```python
from build123d import *

# Parameters (mm, degrees)
F0_W     = 101.6
F0_H     = 101.6
F1_DEPTH = 914.4
F3_DEPTH = 101.6
F4_W     = 101.6
F4_H     = 101.6
F5_DEPTH = 50.8
F6_W     = 50.8
F6_H     = 101.6
F7_DEPTH = 50.8


with BuildPart() as f1:
    # F0 (on Top) → F1 (new body)
    with BuildSketch(Plane.XY):
        Rectangle(F0_W, F0_H)
    extrude(amount=F1_DEPTH)

    # F2 (on face) → F3 (cut)
    with BuildSketch(Plane.XY.offset(914.4)):
        Polygon((-25.4, -50.8), (-50.8, 50.8), (-50.8, -50.8), align=None)
        Polygon((50.8, -50.8), (50.8, 50.8), (25.4, -50.8), align=None)
    extrude(amount=-F3_DEPTH, mode=Mode.SUBTRACT)

    # F4 (on face) → F5 (cut)
    with BuildSketch(Plane.XZ.offset(50.8)):
        with Locations((0, 152.4)):
            Rectangle(F4_W, F4_H)
    extrude(amount=-F5_DEPTH, mode=Mode.SUBTRACT)

    # F6 (on face) → F7 (cut)
    with BuildSketch(Plane(origin=(-50.8, 0, 0), x_dir=(0, -1, 0), z_dir=(-1, 0, 0))):
        with Locations((-25.4, 152.4)):
            Rectangle(F6_W, F6_H)
        with Locations((25.4, 152.4)):
            Rectangle(F6_W, F6_H)
    extrude(amount=-F7_DEPTH, mode=Mode.SUBTRACT)


solid = f1.part
```
Can you work these out from the model? Positions are in its coordinate system, mm. A direction names the side the tool comes from. Give positions to 0.01 mm unless a question says otherwise; leave off trailing zeros. Loops run counter-clockwise (first coordinate to the right, second up) from the corner with the lowest first, then second, coordinate; pieces in that order, holes last. Notation, with made-up numbers: M 2,-8 L 59,-8 A20 cw 59,29 Z; hole C 2,39 d6. An arc over 180 degrees is marked long. One line per item, written item: value.
(1) Suppose I cut it at B-B on x = -37.5. List the corners of the cut face in (y, z) for me.
Returned:
outline: M -50.8,0 L 50.8,0 L 50.8,101.6 L -50.8,101.6 Z; M -50.8,203.2 L 50.8,203.2 L 50.8,914.4 L -2.4,914.4 L -2.4,812.8 L -50.8,812.8 Z
(2) Which directions (+Z, -Z, +X, -X, +Y, -Y) give clear straight access to the entire face, cutting with the end or side of a thin tool? Please do faces 1 (the face through (44, -22, 812.8)), 2 (the face through (0, 26, 153)), 3 (the face through (-44, -22, 812.8)).
Returned:
face 1: +Z, +X, -Y
face 2: -X, +Y, -Y
face 3: +Z, -X, -Y
(3) We'd pull the mould along Z, two halves only. Please class faces 4 (the face through (50.8, -1, 401)), 5 (the face through (-1, 12, 914.4)), 6 (the face through (-12, -11, 101.6)): released by +Z, released by -Z, zero draft, split by the parting line, or undercut.
Returned:
face 4: zero draft
face 5: released by +Z
face 6: undercut
(4) Suppose I cut it at C-C on x = 16. List the corners of the cut face in (y, z) for me.
Returned:
outline: M -50.8,0 L 50.8,0 L 50.8,914.4 L -50.8,914.4 L -50.8,203.2 L 0,203.2 L 0,101.6 L -50.8,101.6 Z
(5) Suppose I cut it at A-A on y = -37. List the corners of the cut face in (x, z) for me.
Returned:
outline: M -50.8,0 L 50.8,0 L 50.8,101.6 L -50.8,101.6 Z; M -50.8,203.2 L 50.8,203.2 L 50.8,812.8 L 28.85,812.8 L 28.85,914.4 L -28.85,914.4 L -28.85,812.8 L -50.8,812.8 Z
(6) I need wall thicknesses on line 1 (Z direction, x = -35.5, y = -20.5); line 2 (Z direction, x = -38, y = 4); line 3 (Y direction, x = 11, z = 112). Which ranges of each line are inside material? Lowest first, please.
Returned:
line 1: 0 to 101.6, 203.2 to 812.8
line 2: 0 to 101.6, 203.2 to 914.4
line 3: 0 to 50.8
